The listing builds one solid part. Answer for the finished solid, in the listing's coordinates (mm). Face numbers are marked on the shaded views. A direction names the side the tool comes from. Round coordinates to 2 decimals unless told otherwise and drop trailing zeros. Write each loop counter-clockwise with the first axis right and the second up, starting at its lowest first coordinate (ties: lowest second). Pieces come first, ordered by that corner, then holes.
from build123d import *

# Parameters (mm, degrees)
F0_W     = 7.7
F0_H     = 1
F0_W_2   = 1
F0_H_2   = 7.7
F1_DEPTH = 9.6
F2_DEPTH = 1.6
F3_START = 8.6
F3_DEPTH = 1
F4_R     = 1.05
F5_DEPTH = 0.6
F6_DEPTH = 1.001


with BuildPart() as f1:
    # F0 (on Top) → F1 (new body)
    with BuildSketch(Plane.XY):
        Polygon((-3.85, 7.85), (-7.85, 7.85), (-7.85, 3.85), (-6.85, 3.85), (-6.85, 6.85), (-3.85, 6.85), align=None)
        with Locations((0, 7.35)):
            Rectangle(F0_W, F0_H)
        with Locations((-7.35, 0)):
            Rectangle(F0_W_2, F0_H_2)
        Polygon((7.85, 7.85), (3.85, 7.85), (3.85, 6.85), (6.85, 6.85), (6.85, 3.85), (7.85, 3.85), align=None)
        Polygon((-6.85, -3.85), (-7.85, -3.85), (-7.85, -7.85), (-3.85, -7.85), (-3.85, -6.85), (-6.85, -6.85), align=None)
        with Locations((7.35, 0)):
            Rectangle(F0_W_2, F0_H_2)
        with Locations((0, -7.35)):
            Rectangle(F0_W, F0_H)
        Polygon((7.85, -7.85), (7.85, -3.85), (6.85, -3.85), (6.85, -6.85), (3.85, -6.85), (3.85, -7.85), align=None)
    extrude(amount=F1_DEPTH)

    # F0 (on Top) → F2 (cut)
    with BuildSketch(Plane.XY):
        with Locations((0, 7.35)):
            Rectangle(F0_W, F0_H)
        with Locations((7.35, 0)):
            Rectangle(F0_W_2, F0_H_2)
        with Locations((0, -7.35)):
            Rectangle(F0_W, F0_H)
        with Locations((-7.35, 0)):
            Rectangle(F0_W_2, F0_H_2)
    extrude(amount=F2_DEPTH, mode=Mode.SUBTRACT)

    # F0 (on Top) → F3 (join)
    with BuildSketch(Plane.XY.offset(F3_START)):
        Polygon((3.85, 6.85), (-3.85, 6.85), (-6.85, 6.85), (-6.85, 3.85), (-6.85, -3.85), (-6.85, -6.85), (-3.85, -6.85), (3.85, -6.85), (6.85, -6.85), (6.85, -3.85), (6.85, 3.85), (6.85, 6.85), align=None)
    extrude(amount=F3_DEPTH)

    # F4 (on face) → F5 (cut)
    with BuildSketch(Plane(origin=(0, 0, 8.6), x_dir=(1, 0, 0), z_dir=(0, 0, -1))):
        with Locations((-5.65, -2.75)):
            Circle(F4_R)
        with Locations((5.65, 2.75)):
            Circle(F4_R)
    extrude(amount=-F5_DEPTH, mode=Mode.SUBTRACT)

    # F4 (on face) → F6 (cut, through all)
    with BuildSketch(Plane(origin=(0, 0, 8.6), x_dir=(1, 0, 0), z_dir=(0, 0, -1))):
        with BuildLine():
            Line((-3.232455532, 6.85), (-1.967544468, 6.85))
            ThreePointArc((-1.967544468, 6.85), (-2.6, 7.05), (-3.232455532, 6.85))
        make_face()
        with BuildLine():
            ThreePointArc((-3.232455532, 6.85), (-3.1070990607, 4.9738593633), (-1.5, 5.95))
            ThreePointArc((-1.5, 5.95), (-1.6238593633, 6.4570990607), (-1.967544468, 6.85))
            Line((-1.967544468, 6.85), (-3.232455532, 6.85))
        make_face()
        with BuildLine():
            ThreePointArc((0.632455532, 6.85), (0, 7.05), (-0.632455532, 6.85))
            Line((-0.632455532, 6.85), (0.632455532, 6.85))
        make_face()
        with BuildLine():
            Line((0.632455532, 6.85), (-0.632455532, 6.85))
            ThreePointArc((-0.632455532, 6.85), (-0.5070990607, 4.9738593633), (1.1, 5.95))
            ThreePointArc((1.1, 5.95), (0.9761406367, 6.4570990607), (0.632455532, 6.85))
        make_face()
        with BuildLine():
            ThreePointArc((3.232455532, 6.85), (2.6, 7.05), (1.967544468, 6.85))
            Line((1.967544468, 6.85), (3.232455532, 6.85))
        make_face()
        with BuildLine():
            Line((3.232455532, 6.85), (1.967544468, 6.85))
            ThreePointArc((1.967544468, 6.85), (2.0929009393, 4.9738593633), (3.7, 5.95))
            ThreePointArc((3.7, 5.95), (3.5761406367, 6.4570990607), (3.232455532, 6.85))
        make_face()
    extrude(amount=-F6_DEPTH, mode=Mode.SUBTRACT)


solid = f1.part
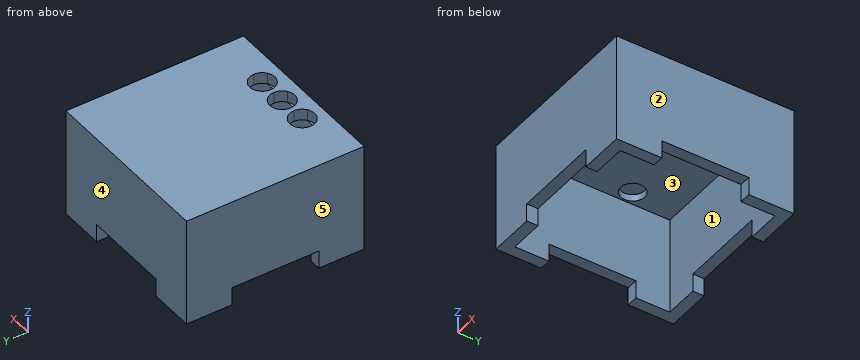
1. A tool of negligible diameter and unlimited length cuts with its end or side. For the marked faces 1 and 2, from which of +Z, -Z, +X, -X, +Y, -Y can it reach the whole face along a straight path? Write none if from no direction.
Geometry says:
face 1: -Z
face 2: +Z, -Z, +X, +Y, -Y
2. Section D-D on z = 9 is taken. Determine the outline of the cut face in (x, y), plus the area to 3 significant figures.
Geometry says:
outline: (-7.85, -7.85) - (7.85, -7.85) - (7.85, 7.85) - (-7.85, 7.85) - close; hole circle Ø2.1 at (-5.65, 2.75); hole circle Ø2.2 at (-2.6, -5.95); hole circle Ø2.2 at (0, -5.95); hole circle Ø2.2 at (2.6, -5.95); hole circle Ø2.1 at (5.65, -2.75)
area: 228 mm2
3. Straight lines are drawn through the part: line 1 along X through (y, z) = (-5.95, 9.25); line 2 along Y through (x, z) = (-5.25, 7.5); line 3 along X through (y, z) = (-2.75, 9.05). For each, find the intervals that lie inside material, in ascending order.
Geometry says:
line 1: x = -7.85 to -3.7, -1.5 to -1.1, 1.1 to 1.5, 3.7 to 7.85
line 2: y = -7.85 to -6.85, 6.85 to 7.85
line 3: x = -7.85 to 4.6, 6.7 to 7.85
4. For a pull along X with two mould halves and no side action, classify the marked faces 3, 4 and 5 as released by +X, released by -X, zero draft, split by the parting line, or undercut.
Geometry says:
face 3: undercut
face 4: zero draft
face 5: released by -X
5. Section C-C on y = 2.75 is taken. Determine the outline of the cut face in (x, z).
Geometry says:
outline: (-7.85, 1.6) - (-6.85, 1.6) - (-6.85, 8.6) - (-6.7, 8.6) - (-6.7, 9.2) - (-4.6, 9.2) - (-4.6, 8.6) - (6.85, 8.6) - (6.85, 1.6) - (7.85, 1.6) - (7.85, 9.6) - (-7.85, 9.6) - close
6. Section A-A on z = 1 is taken. Determine the outline of the cut face in (x, y), plus the area to 3 significant figures.
Geometry says:
outline: (-7.85, -7.85) - (-3.85, -7.85) - (-3.85, -6.85) - (-6.85, -6.85) - (-6.85, -3.85) - (-7.85, -3.85) - close; (-7.85, 3.85) - (-6.85, 3.85) - (-6.85, 6.85) - (-3.85, 6.85) - (-3.85, 7.85) - (-7.85, 7.85) - close; (3.85, -7.85) - (7.85, -7.85) - (7.85, -3.85) - (6.85, -3.85) - (6.85, -6.85) - (3.85, -6.85) - close; (3.85, 6.85) - (6.85, 6.85) - (6.85, 3.85) - (7.85, 3.85) - (7.85, 7.85) - (3.85, 7.85) - close
area: 28.0 mm2
7. Given pin 1 (1.5 mm diameter, centred on x = -5.5, y = 6, fed in from -Z); pin 2 (1 mm diameter, centred on x = -5.5, y = 3, fed in from -Z); pin 3 (0.5 mm diameter, centred on x = -7.5, y = -0.5, fed in from -Z), each flat-ended and moving along its own axis, determine where each tip first touches the part or whether it passes through.
Geometry says:
pin 1: stops at z = 8.6
pin 2: stops at z = 9.2
pin 3: stops at z = 1.6
8. Section B-B on x = 2.6 is taken. Determine the outline of the cut face in (y, z).
Geometry says:
outline: (-7.85, 1.6) - (-6.85, 1.6) - (-6.85, 8.6) - (-7.05, 8.6) - (-7.05, 9.6) - (-7.85, 9.6) - close; (-4.85, 8.6) - (6.85, 8.6) - (6.85, 1.6) - (7.85, 1.6) - (7.85, 9.6) - (-4.85, 9.6) - close
